Input: part model. Units: mm. Frame: model coordinates. Give positions to 0.01 mm unless a question says otherwise; leave off trailing zeros. Loops run counter-clockwise (first coordinate to the right, second up) from the corner with the lowest first, then second, coordinate; pieces in that order, holes last. Notation, with made-up numbers: (31.5, 1.5) - (70.5, 1.5) arc R16 cw to (70.5, 12.5) - close; hole circle Ø4 at (18, 74.5). An arc over 180 degrees is marked (long way). One line per question, with ' | ' between items. Start each with the question number.
from build123d import *

# Parameters (mm, degrees)
SKETCH2_R           = 2
BOSS_EXTRUDE1_DEPTH = 11.6
SKETCH3_R           = 4
BOSS_EXTRUDE2_DEPTH = 0.3
SKETCH4_R           = 8
BOSS_EXTRUDE3_DEPTH = 0.7
SKETCH5_R           = 1.5
CUT_EXTRUDE1_DEPTH  = 8.5
SKETCH6_R           = 1.5
CUT_EXTRUDE2_DEPTH  = 17.419805115
CHAMFER1_SIZE       = 0.1


with BuildPart() as part:
    # Sketch2 → Boss-Extrude1 (new body)
    with BuildSketch(Plane(origin=(0, 0, 0), x_dir=(1, 0, 0), z_dir=(0, 1, 0))):
        with Locations(Location((0, 0, 0), (0, 0, 270))):
            Circle(SKETCH2_R)
    extrude(amount=BOSS_EXTRUDE1_DEPTH)

    # Sketch3 → Boss-Extrude2 (add)
    with BuildSketch(Plane(origin=(0, 11.6, 0), x_dir=(1, 0, 0), z_dir=(0, 1, 0))):
        with Locations(Location((0, 0, 0), (0, 0, 270))):
            Circle(SKETCH3_R)
    extrude(amount=BOSS_EXTRUDE2_DEPTH)

    # Sketch4 → Boss-Extrude3 (add)
    with BuildSketch(Plane(origin=(0, 11.9, 0), x_dir=(1, 0, 0), z_dir=(0, 1, 0))):
        with Locations(Location((0, 0, 0), (0, 0, 270))):
            Circle(SKETCH4_R)
    extrude(amount=BOSS_EXTRUDE3_DEPTH)

    # Sketch5 → Cut-Extrude1 (cut)
    with BuildSketch(Plane.XZ):
        with Locations(Location((0, 0, 0), (0, 0, 270))):
            Circle(SKETCH5_R)
    extrude(amount=-CUT_EXTRUDE1_DEPTH, mode=Mode.SUBTRACT)

    # Sketch6 → Cut-Extrude2 (cut, through all)
    with BuildSketch(Plane.XZ.offset(-11.9)):
        with Locations(Location((0, -6, 0), (0, 0, 270))):
            Circle(SKETCH6_R)
    extrude(amount=-CUT_EXTRUDE2_DEPTH, mode=Mode.SUBTRACT)

    # Chamfer1
    chamfer1_edges = [part.edges().sort_by_distance(p)[0] for p in [
        (0, 12.6, -8),
        (0, 11.9, -8),
    ]]
    chamfer(chamfer1_edges, length=CHAMFER1_SIZE)


solid = part.part
Q1. First-contact query: pin 1 (4 mm diameter, centred on y = 11, z = 2.5, fed in from -X); pin 2 (6 mm diameter, centred on y = 4.5, z = -4.5, fed in from +X); pin 3 (1.5 mm diameter, centred on x = -0.5, z = 0, fed in from -Y). Flat tips, straight axial feed; report the tip coordinate or a pass-through.
Q2. Section D-D, the plane y = 11. Output: boundary loops of the cut face in (x, z), plus the area to 3 significant figures.
Q3. Section C-C, the plane y = 2.25. Output: boundary loops of the cut face in (x, z), plus the area to 3 significant figures.
Q4. Section A-A, the plane x = 0. Output: boundary loops of the cut face in (y, z).
Q5. Section B-B, the plane z = 0. Output: boundary loops of the cut face in (x, y).
Q6. Line query: L1, parallel to X at y = 1.5, z = 0; L2, parallel to Y at x = -4.75, z = -2.5; L3, parallel to Y at x = -1.5, z = -2.75. Output: solid intervals per line, ascending. Write a range as from..to.
Q7. Draft query along X for faces 1 (the face through (0.07, 12.25, -4.5)), 2 (the face through (0, 12.6, 0)), 3 (the face through (-7.81, 12.25, -1.73)). Return one class per face: +X half, -X half, draft (parallel to the pull), parting line (faces both ways), or undercut.
Solved:
1) pin 1: stops at x = -7.96 | pin 2: stops at x = 1.32 | pin 3: stops at y = 8.5
2) outline: circle Ø4 at (0, 0) | area: 12.6 mm²
3) outline: circle Ø4 at (0, 0); hole circle Ø3 at (0, 0) | area: 5.50 mm²
4) outline: (0, -2) - (11.6, -2) - (11.6, -4) - (11.9, -4) - (11.9, -4.5) - (12.6, -4.5) - (12.6, 7.9) - (12.5, 8) - (12, 8) - (11.9, 7.9) - (11.9, 4) - (11.6, 4) - (11.6, 2) - (0, 2) - (0, 1.5) - (8.5, 1.5) - (8.5, -1.5) - (0, -1.5) - close; (11.9, -7.9) - (12, -8) - (12.5, -8) - (12.6, -7.9) - (12.6, -7.5) - (11.9, -7.5) - close
5) outline: (-8, 12) - (-7.9, 11.9) - (-4, 11.9) - (-4, 11.6) - (-2, 11.6) - (-2, 0) - (-1.5, 0) - (-1.5, 8.5) - (1.5, 8.5) - (1.5, 0) - (2, 0) - (2, 11.6) - (4, 11.6) - (4, 11.9) - (7.9, 11.9) - (8, 12) - (8, 12.5) - (7.9, 12.6) - (-7.9, 12.6) - (-8, 12.5) - close
6) L1: x = -2..-1.5, 1.5..2 | L2: y = 11.9..12.6 | L3: y = 11.6..12.6
7) face 1: undercut | face 2: draft | face 3: parting line
